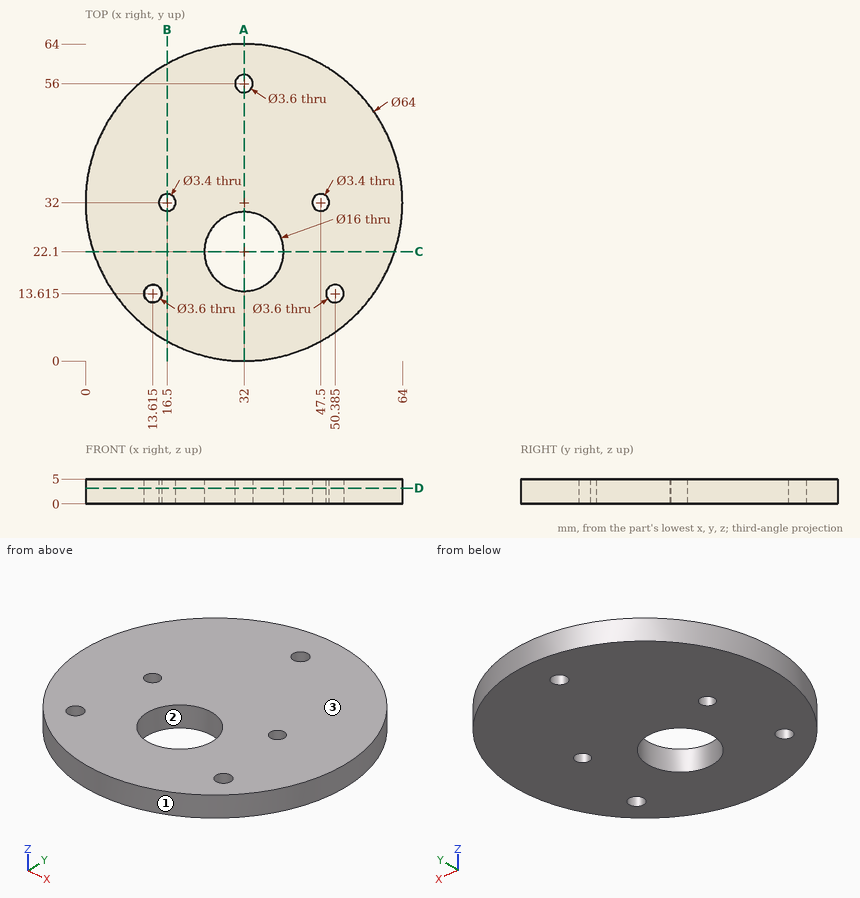
Geometry check sheet. Reference: drawing and pictorial views, mm from the part's lowest x, y, z. Give positions to 0.01 mm unless a question says otherwise; leave off trailing zeros. Write each loop counter-clockwise with the first axis right and the second up, starting at its lowest first coordinate (ties: lowest second). Pieces come first, ordered by that corner, then holes.
Item 1: Scan lines: L1, parallel to X at y = 32.5, z = 2.5 (1 decimal); L2, parallel to X at y = 26.5, z = 0.35; L3, parallel to Y at x = 37.5, z = 1.95. Record each from-to range of solid material in increasing order.
Item 2: Cross-section at C-C (y = 22.1). Enter the section's corners in (x, z).
Item 3: Cross-section at A-A (x = 32). Enter the section's corners in (y, z).
Item 4: Gauge pin test, flat ends, axial feed: pin 1 (2 mm diameter, centred on x = 38.5, z = 2.5, fed in from -Y); pin 2 (4.5 mm diameter, centred on x = 16.5, y = 32, fed in from +Z); pin 3 (3 mm diameter, centred on x = 32, y = 56, fed in from +Z); pin 4 (1 mm diameter, centred on y = 22.5, z = 1.5, fed in from +X). Record the tip position at first contact, or that the pin passes through.
Item 5: Cross-section at B-B (x = 16.5). Enter the section's corners in (y, z).
Item 6: Draft check along Y on the marked faces 1, 2 and 3. Enter one of: released by +Y, released by -Y, zero draft, split by the parting line, or undercut.
Item 7: Cross-section at D-D (z = 3.15). Enter the section's corners in (x, y) (1 decimal), and give its area (3 significant figures).
Report:
1. L1: x = 0 to 14.9, 18.1 to 45.9, 49.1 to 64
1. L2: x = 0.48 to 25.32, 38.68 to 63.52
1. L3: y = 0.48 to 16.29, 27.91 to 63.52
2. outline: (1.57, 0) - (24, 0) - (24, 5) - (1.57, 5) - close; (40, 0) - (62.43, 0) - (62.43, 5) - (40, 5) - close
3. outline: (0, 0) - (14.1, 0) - (14.1, 5) - (0, 5) - close; (30.1, 0) - (54.2, 0) - (54.2, 5) - (30.1, 5) - close; (57.8, 0) - (64, 0) - (64, 5) - (57.8, 5) - close
4. pin 1: stops at y = 0.48
4. pin 2: stops at z = 5
4. pin 3: passes through
4. pin 4: stops at x = 62.71
5. outline: (4, 0) - (30.3, 0) - (30.3, 5) - (4, 5) - close; (33.7, 0) - (60, 0) - (60, 5) - (33.7, 5) - close
6. face 1: split by the parting line
6. face 2: undercut
6. face 3: zero draft
7. outline: circle Ø64 at (32, 32); hole circle Ø3.6 at (13.6, 13.6); hole circle Ø3.4 at (16.5, 32); hole circle Ø16 at (32, 22.1); hole circle Ø3.6 at (32, 56); hole circle Ø3.4 at (47.5, 32); hole circle Ø3.6 at (50.4, 13.6)
7. area: 2,970 mm2
